```python
from build123d import *

# Parameters (mm, degrees)
BOSS_EXTRUDE1_DEPTH  = 2.54
BOSS_EXTRUDE2_START  = -288.5
BOSS_EXTRUDE2_DEPTH  = 36.75
BOSS_EXTRUDE3_START  = -36.75
SKETCH4_3_W          = 2.2
SKETCH4_3_H          = 10
BOSS_EXTRUDE3_DEPTH  = 36.75
CUT_EXTRUDE1_DEPTH   = 161.627285976
SKETCH2_W            = 3.357693748
SKETCH2_H            = 2.2
BOSS_EXTRUDE4_DEPTH  = 5
FILLET1_R            = 4.5
FILLET2_R            = 2.5
BOSS_EXTRUDE5_REACH  = 154.276
SKETCH2_3_W          = 3.357693748
SKETCH2_3_H          = 2
BOSS_EXTRUDE6_REACH  = 154.276
CUT_EXTRUDE8_DEPTH   = 293.931412621
FILLET3_R            = 2.5
CUT_EXTRUDE2_DEPTH   = 2.54
CUT_EXTRUDE3_DEPTH   = 1.54
CUT_EXTRUDE4_DEPTH   = 2.54
CUT_EXTRUDE5_DEPTH   = 1.54
SKETCH9_W            = 8.6
SKETCH9_H            = 4.2
SKETCH9_W_2          = 7.6
CUT_EXTRUDE6_DEPTH   = 1.2
SKETCH10_W           = 6.75
SKETCH10_H           = 4
SKETCH10_W_2         = 8
CUT_EXTRUDE7_DEPTH   = 1.2
SKETCH12_W           = 6
SKETCH12_H           = 5
SKETCH12_H_2         = 7
BOSS_EXTRUDE7_DEPTH  = 2
DRAFT1_ANGLE         = 60
SKETCH13_W           = 5
SKETCH13_H           = 1.75
BOSS_EXTRUDE8_DEPTH  = 4
SKETCH14_W           = 4
SKETCH14_H           = 5
BOSS_EXTRUDE9_DEPTH  = 1.5
SKETCH15_W           = 1.75
SKETCH15_H           = 5
BOSS_EXTRUDE10_DEPTH = 4.25
DRAFT2_ANGLE         = 5
DRAFT3_ANGLE         = 5
SKETCH16_W           = 2.125
SKETCH16_H           = 7
BOSS_EXTRUDE11_DEPTH = 1
CHAMFER1_SIZE        = 1
CHAMFER1_SIZE2       = 2
SKETCH17_W           = 0.5
SKETCH17_H           = 10
CUT_EXTRUDE9_DEPTH   = 1


with BuildPart() as part:
    # Sketch1 → Boss-Extrude1 (new body)
    with BuildSketch(Plane(origin=(0, 0, 0), x_dir=(0, 1, 0), z_dir=(0, 0, 1))):
        Polygon((-107.5, 27), (-144.25, 27), (-144.25, -27), (144.25, -27), (144.25, 27), (107.5, 27), (107.5, 2), (-107.5, 2), align=None)
    extrude(amount=BOSS_EXTRUDE1_DEPTH)

    # Sketch4 → Boss-Extrude2 (add)
    with BuildSketch(Plane.XZ.offset(144.25).offset(BOSS_EXTRUDE2_START)):
        with BuildLine():
            Line((-30.446882411, 8.073506155), (-27.715620382, 1.676171354))
            Line((-27.715620382, 1.676171354), (-27, 1.98169652))
            Line((-27, 1.98169652), (-27, 2.54))
            Line((-27, 2.54), (-25.692306252, 2.54))
            Line((-25.692306252, 2.54), (-28.246882411, 8.523489974))
            ThreePointArc((-28.246882411, 8.523489974), (-28.84716347, 10.446090622), (-29.05, 12.449983819))
            Line((-29.05, 12.449983819), (-29.05, 30))
            Line((-29.05, 30), (-31.25, 30))
            Line((-31.25, 30), (-31.25, 12))
            ThreePointArc((-31.25, 12), (-31.04716347, 9.996106803), (-30.446882411, 8.073506155))
        make_face()
        Polygon((-27.715620382, 1.676171354), (-27, 0), (-27, 1.98169652), align=None)
    extrude(amount=BOSS_EXTRUDE2_DEPTH)

    # Sketch4<3> → Boss-Extrude3 (add)
    with BuildSketch(Plane.XZ.offset(144.25).offset(BOSS_EXTRUDE3_START)):
        with BuildLine():
            Line((-30.446882411, 8.073506155), (-27.715620382, 1.676171354))
            Line((-27.715620382, 1.676171354), (-27, 1.98169652))
            Line((-27, 1.98169652), (-27, 2.54))
            Line((-27, 2.54), (-25.692306252, 2.54))
            Line((-25.692306252, 2.54), (-28.246882411, 8.523489974))
            ThreePointArc((-28.246882411, 8.523489974), (-28.84716347, 10.446090622), (-29.05, 12.449983819))
            Line((-29.05, 12.449983819), (-29.05, 30))
            Line((-29.05, 30), (-31.25, 30))
            Line((-31.25, 30), (-31.25, 12))
            ThreePointArc((-31.25, 12), (-31.04716347, 9.996106803), (-30.446882411, 8.073506155))
        make_face()
        with Locations((-30.15, 35)):
            Rectangle(SKETCH4_3_W, SKETCH4_3_H)
        Polygon((-27.715620382, 1.676171354), (-27, 0), (-27, 1.98169652), align=None)
    extrude(amount=BOSS_EXTRUDE3_DEPTH)

    # Sketch5 → Cut-Extrude1 (cut, through all)
    with BuildSketch(Plane(origin=(-31.25, 0, 0), x_dir=(0, -1, 0), z_dir=(-1, 0, 0))):
        Polygon((-134.25, 30), (-134.25, 23), (-144.25, 11), (-144.25, 30), align=None)
        Polygon((144.25, 11), (134.25, 23), (134.25, 40), (144.25, 40), align=None)
    extrude(amount=-CUT_EXTRUDE1_DEPTH, mode=Mode.SUBTRACT)

    # Sketch2 → Boss-Extrude4 (add)
    with BuildSketch(Plane.XY.offset(2.54)):
        Polygon((0.2, 109.7), (-25.692306252, 109.7), (-25.692306252, 107.5), (-2, 107.5), (-2, -107.5), (-25.692306252, -107.5), (-25.692306252, -109.7), (0.2, -109.7), align=None)
        with Locations((-27.371153126, -108.6)):
            Rectangle(SKETCH2_W, SKETCH2_H)
        with Locations((-27.371153126, 108.6)):
            Rectangle(SKETCH2_W, SKETCH2_H)
    extrude(amount=BOSS_EXTRUDE4_DEPTH)

    # Fillet1
    fillet1_edges = [part.edges().sort_by_distance(p)[0] for p in [
        (0.2, 109.7, 5.04),
        (0.2, -109.7, 5.04),
    ]]
    fillet(fillet1_edges, radius=FILLET1_R)

    # Fillet2
    fillet2_edges = [part.edges().sort_by_distance(p)[0] for p in [
        (-2, -107.5, 3.77),
        (-2, 107.5, 3.77),
    ]]
    fillet(fillet2_edges, radius=FILLET2_R)

    # Boss-Extrude5: up to this face of the body (flat: up to its plane)
    boss_extrude5_end = Plane(part.part.faces().sort_by_distance((-30.15, -120.875, 40))[0])
    # Sketch2<3> → Boss-Extrude5 (add, up to the picked face)
    with BuildSketch(Plane.XY.offset(2.54), mode=Mode.PRIVATE) as boss_extrude5_sk1:
        Polygon((27, -139.25), (27, -136.71), (-15, -136.71), (-15, -132.25), (-25.692306252, -132.25), (-25.692306252, -134.25), (-17.54, -134.25), (-17.54, -139.25), align=None)
    boss_extrude5_tool1 = split(extrude(boss_extrude5_sk1.sketch, amount=BOSS_EXTRUDE5_REACH, mode=Mode.PRIVATE), bisect_by=boss_extrude5_end, keep=Keep.BOTH, mode=Mode.PRIVATE)
    # Sketch2<3> → Boss-Extrude5 (add, up to the picked face)
    with BuildSketch(Plane.XY.offset(2.54), mode=Mode.PRIVATE) as boss_extrude5_sk2:
        with Locations((-27.371153126, -133.25)):
            Rectangle(SKETCH2_3_W, SKETCH2_3_H)
    boss_extrude5_tool2 = split(extrude(boss_extrude5_sk2.sketch, amount=BOSS_EXTRUDE5_REACH, mode=Mode.PRIVATE), bisect_by=boss_extrude5_end, keep=Keep.BOTH, mode=Mode.PRIVATE)
    add(boss_extrude5_tool1.solids().sort_by(Axis((-0.011676, -137.150458, 2.54), (0, 0, 1)))[0])
    add(boss_extrude5_tool2.solids().sort_by(Axis((-27.371153, -133.25, 2.54), (0, 0, 1)))[0])

    # Boss-Extrude6: up to this face of the body (flat: up to its plane)
    boss_extrude6_end = Plane(part.part.faces().sort_by_distance((-30.15, 120.875, 30))[0])
    # Sketch2<4> → Boss-Extrude6 (add, up to the picked face)
    with BuildSketch(Plane.XY.offset(2.54), mode=Mode.PRIVATE) as boss_extrude6_sk1:
        Polygon((-29.05, 134.25), (-15, 134.25), (-15, 139.05), (27, 139.05), (27, 136.51), (-12.46, 136.51), (-12.46, 132.25), (-29.05, 132.25), align=None)
    boss_extrude6_tool1 = split(extrude(boss_extrude6_sk1.sketch, amount=BOSS_EXTRUDE6_REACH, mode=Mode.PRIVATE), bisect_by=boss_extrude6_end, keep=Keep.BOTH, mode=Mode.PRIVATE)
    add(boss_extrude6_tool1.solids().sort_by(Axis((-0.874906, 136.653064, 2.54), (0, 0, 1)))[0])

    # Sketch11 → Cut-Extrude8 (cut, through all)
    with BuildSketch(Plane.XZ.offset(144.25)):
        Polygon((-27, 0), (-30.446882411, 8.073506155), (-30.446882411, 0), align=None)
    extrude(amount=-CUT_EXTRUDE8_DEPTH, mode=Mode.SUBTRACT)

    # Fillet3
    fillet3_edges = [part.edges().sort_by_distance(p)[0] for p in [
        (-27, 125.875, 0),
        (-27, -125.875, 0),
    ]]
    fillet(fillet3_edges, radius=FILLET3_R)

    # Sketch7 → Cut-Extrude2 (cut)
    with BuildSketch(Plane.XZ.offset(139.25)):
        with BuildLine():
            ThreePointArc((25, 36.2), (26.414213562, 35.614213562), (27, 34.2))
            Line((27, 34.2), (27, 36.2))
            Line((27, 36.2), (27, 40))
            Line((27, 40), (-12, 40))
            Line((-12, 40), (-12, 36.2))
            Line((-12, 36.2), (25, 36.2))
        make_face()
    extrude(amount=-CUT_EXTRUDE2_DEPTH, mode=Mode.SUBTRACT)

    # Sketch7<3> → Cut-Extrude3 (cut)
    with BuildSketch(Plane.XZ.offset(139.25)):
        with BuildLine():
            Line((-10, 32.2), (27, 32.2))
            Line((27, 32.2), (27, 34.2))
            ThreePointArc((27, 34.2), (26.414213562, 35.614213562), (25, 36.2))
            Line((25, 36.2), (-12, 36.2))
            Line((-12, 36.2), (-12, 34.2))
            ThreePointArc((-12, 34.2), (-11.414213562, 32.785786438), (-10, 32.2))
        make_face()
    extrude(amount=-CUT_EXTRUDE3_DEPTH, mode=Mode.SUBTRACT)

    # Sketch8 → Cut-Extrude4 (cut)
    with BuildSketch(Plane(origin=(0, 139.05, 0), x_dir=(-1, 0, 0), z_dir=(0, 1, 0))):
        with BuildLine():
            Line((12, 26.2), (12, 30))
            Line((12, 30), (-27, 30))
            Line((-27, 30), (-27, 23.2))
            ThreePointArc((-27, 23.2), (-26.121320344, 25.321320344), (-24, 26.2))
            Line((-24, 26.2), (12, 26.2))
        make_face()
    extrude(amount=-CUT_EXTRUDE4_DEPTH, mode=Mode.SUBTRACT)

    # Sketch8<3> → Cut-Extrude5 (cut)
    with BuildSketch(Plane(origin=(0, 139.05, 0), x_dir=(-1, 0, 0), z_dir=(0, 1, 0))):
        with BuildLine():
            Line((12, 25.2), (12, 26.2))
            Line((12, 26.2), (-24, 26.2))
            ThreePointArc((-24, 26.2), (-26.121320344, 25.321320344), (-27, 23.2))
            Line((-27, 23.2), (-27, 22.2))
            Line((-27, 22.2), (9, 22.2))
            ThreePointArc((9, 22.2), (11.121320344, 23.078679656), (12, 25.2))
        make_face()
    extrude(amount=-CUT_EXTRUDE5_DEPTH, mode=Mode.SUBTRACT)

    # Sketch9 → Cut-Extrude6 (cut)
    with BuildSketch(Plane.YZ.offset(-29.05)):
        with Locations((-127.95, 37.9)):
            Rectangle(SKETCH9_W, SKETCH9_H)
        with Locations((-111.3, 37.9)):
            Rectangle(SKETCH9_W_2, SKETCH9_H)
    extrude(amount=-CUT_EXTRUDE6_DEPTH, mode=Mode.SUBTRACT)

    # Sketch10 → Cut-Extrude7 (cut)
    with BuildSketch(Plane.YZ.offset(-29.05)):
        with Locations((110.875, 28)):
            Rectangle(SKETCH10_W, SKETCH10_H)
        with Locations((128.25, 28)):
            Rectangle(SKETCH10_W_2, SKETCH10_H)
    extrude(amount=-CUT_EXTRUDE7_DEPTH, mode=Mode.SUBTRACT)

    # Sketch12 → Boss-Extrude7 (add)
    with BuildSketch(Plane.XY.offset(2.54)):
        with Locations((28.25, -120.5)):
            Rectangle(SKETCH12_W, SKETCH12_H)
        with Locations((28.25, -5)):
            Rectangle(SKETCH12_W, SKETCH12_H_2)
        with Locations((28.25, 119.5)):
            Rectangle(SKETCH12_W, SKETCH12_H)
    extrude(amount=BOSS_EXTRUDE7_DEPTH)

    # Draft1
    draft1_faces = [part.faces().sort_by_distance(p)[0] for p in [
        (25.25, -120.5, 3.54),
        (25.25, -5, 3.54),
        (25.25, 119.5, 3.54),
    ]]
    draft(draft1_faces, Plane.XY.offset(4.54), DRAFT1_ANGLE)

    # Sketch13 → Boss-Extrude8 (add)
    with BuildSketch(Plane.YZ.offset(-29.05)):
        with Locations((-119.375, 39.125)):
            Rectangle(SKETCH13_W, SKETCH13_H)
        with Locations((119.25, 29.125)):
            Rectangle(SKETCH13_W, SKETCH13_H)
    extrude(amount=BOSS_EXTRUDE8_DEPTH)

    # Sketch14 → Boss-Extrude9 (add)
    with BuildSketch(Plane.YZ.offset(25.5)):
        with Locations((134.51, 19.7)):
            Rectangle(SKETCH14_W, SKETCH14_H)
        with Locations((-134.71, 29.7)):
            Rectangle(SKETCH14_W, SKETCH14_H)
    extrude(amount=BOSS_EXTRUDE9_DEPTH)

    # Sketch15 → Boss-Extrude10 (add)
    with BuildSketch(Plane.YZ.offset(27)):
        with Locations((-133.585, 29.7)):
            Rectangle(SKETCH15_W, SKETCH15_H)
        with Locations((133.385, 19.7)):
            Rectangle(SKETCH15_W, SKETCH15_H)
    extrude(amount=BOSS_EXTRUDE10_DEPTH)

    # Draft2
    draft2_faces = [part.faces().sort_by_distance(p)[0] for p in [
        (-2.659119817, 140.861198407, 2.54),
    ]]
    draft(draft2_faces, Plane(origin=(0, 139.05, 86.460982103), x_dir=(0, 0, 1), z_dir=(0, 1, 0)), DRAFT2_ANGLE)

    # Draft3
    draft3_faces = [part.faces().sort_by_distance(p)[0] for p in [
        (-2.330014026, -141.080071643, 2.54),
    ]]
    draft(draft3_faces, Plane(origin=(0, -139.25, 96.485418472), x_dir=(0, 0, -1), z_dir=(0, -1, 0)), DRAFT3_ANGLE)

    # Sketch16 → Boss-Extrude11 (add)
    with BuildSketch(Plane(origin=(0, 0, 2.54), x_dir=(1, 0, 0), z_dir=(0, 0, -1))):
        with Locations((30.1875, 5)):
            Rectangle(SKETCH16_W, SKETCH16_H)
    extrude(amount=BOSS_EXTRUDE11_DEPTH)

    # Chamfer1
    chamfer1_edges = [part.edges().sort_by_distance(p)[0] for p in [
        (31.25, -5, 1.54),
    ]]
    chamfer1_side = [part.faces().sort_by_distance(p)[0] for p in [
        (31.25, -5, 3.04),
    ]]
    chamfer(chamfer1_edges, length=CHAMFER1_SIZE, length2=CHAMFER1_SIZE2, reference=chamfer1_side[0])

    # Sketch17 → Cut-Extrude9 (cut)
    with BuildSketch(Plane(origin=(0, 0, 0), x_dir=(1, 0, 0), z_dir=(0, 0, -1))):
        Polygon((18, 0), (19.8, -5), (19.8, 5), align=None)
        with Locations((21.25, 0)):
            Rectangle(SKETCH17_W, SKETCH17_H)
        with Locations((22.75, 0)):
            Rectangle(SKETCH17_W, SKETCH17_H)
    extrude(amount=-CUT_EXTRUDE9_DEPTH, mode=Mode.SUBTRACT)


solid = part.part
```
The model under review builds one solid part; all positions refer to its coordinate system, in mm. A direction names the side the tool comes from. Coordinates: 2 decimals unless noted, no trailing zeros. Order: outer loops, then holes, each group sorted by start corner. A loop starts at its lowest first (then second) coordinate and runs counter-clockwise, first axis right, second up. Notation, with made-up numbers: (45, 42.25) -> (60, 42.25) arc R25 ccw to (60, 56.25) -> close; hole circle Ø7 at (7, -39.5). An arc over 180 degrees is marked (long way). Answer in a Markdown table with one row per item. Add a question column.
Item 1: Clearance check with flat-ended pins moving along their axes: pin 1 (4 mm diameter, centred on y = 23.5, z = 2, fed in from -X); pin 2 (10 mm diameter, centred on x = 18.5, y = -52, fed in from +Z); pin 3 (4 mm diameter, centred on x = -4, z = 27.5, fed in from -Y). State where each tip first meets the part, or that it passes through.
Item 2: To check wall thickness, follow probe 1 along Y at (x, z) = (-4, 7); probe 2 along Y at (x, z) = (-12, 14); probe 3 along Y at (x, z) = (-16, 19.5). State the ranges of each line that lie inside material, in increasing order.
Item 3: Mouldability with a two-part tool opening along Z and no side actions: class faces 6 (the flat face through (-29.05, 120, 19)), 7 (the flat face through (-16, 109.7, 5)), 8 (the flat face through (28, 120, 4.54)) as +Z half, -Z half, draft (parallel to the pull), parting line (faces both ways), or undercut.
Item 4: We need section A-A on x = -21. Write out the cut boundary in (y, z).
Item 5: We need section B-B on y = -76. Write out the cut boundary in (x, z).
Item 6: Machinability: for faces 1 (the flat face through (-26.853, 139.32, 5.259)), 2 (the flat face through (28, -120, 4.54)), 3 (the flat face through (6, 139.05, 13)), 4 (the flat face through (-29.05, -138, 16)), 5 (the flat face through (-30.113, 139.18, 17.084)), which of the approach directions +Z, -Z, +X, -X, +Y, -Y give a long, thin tool a straight path to every point of the face, cutting with its end or side? Answer none if there is none.
Final values:
| question | item | result |
|---|---|---|
| 1 | pin 1 | stops at x = -2 |
| 1 | pin 2 | stops at z = 2.54 |
| 1 | pin 3 | stops at y = -139.25 |
| 2 | probe 1 | y = -139.25 to -136.71, -109.69 to -107.45, 107.45 to 109.69, 136.51 to 139.05 |
| 2 | probe 2 | y = -139.25 to -136.71, 136.51 to 139.05 |
| 2 | probe 3 | y = -139.25 to -132.25, 132.25 to 134.25 |
| 3 | face 6 | undercut |
| 3 | face 7 | draft |
| 3 | face 8 | +Z half |
| 4 | outline | (-144.25, 0) -> (-107.5, 0) -> (-107.5, 7.54) -> (-109.7, 7.54) -> (-109.7, 2.54) -> (-132.25, 2.54) -> (-132.25, 40) -> (-134.25, 40) -> (-134.25, 2.98) -> (-144.25, 2.1) -> close; (107.5, 0) -> (144.25, 0) -> (144.25, 2.09) -> (134.25, 2.96) -> (134.25, 30) -> (132.25, 30) -> (132.25, 2.54) -> (109.7, 2.54) -> (109.7, 7.54) -> (107.5, 7.54) -> close |
| 5 | outline | (-2, 0) -> (27, 0) -> (27, 2.54) -> (0.2, 2.54) -> (0.2, 7.54) -> (-2, 7.54) -> close |
| 6 | face 1 | +Z, +Y |
| 6 | face 2 | +Z, +X |
| 6 | face 3 | +Z, +X, +Y |
| 6 | face 4 | +Z, -Y |
| 6 | face 5 | +Z, -X, +Y |
